Can you work these out from the model? Positions are in its coordinate system, mm. A direction names the side the tool comes from. Round coordinates to 2 decimals unless told otherwise and drop trailing zeros. Order: outer loops, then holes, each group sorted by start corner. A loop starts at its lowest first (then second) coordinate and runs counter-clockwise, first axis right, second up. Notation, with made-up numbers: (89, -27.5) -> (141, -27.5) arc R15 cw to (141, -15.5) -> close; hole circle Ø3 at (55.5, 47.5). An arc over 180 degrees is marked (long way). Use a Markdown table: item, result. Add a question column.
Q1. If we section it at A-A on y = 0: Give the number of separate pieces and of enclosed holes in the cut face, plus the area to 3 significant figures.
Q2. I'm going to push flat-ended pins straight in: pin 1 Ø3 at (y, z) = (2.5, 10) entering from +X; pin 2 Ø2 at (x, z) = (-7, 4) entering from +Y; pin 3 Ø5 at (x, z) = (-4, 11.5) entering from +Y; pin 4 Ø3 at (x, y) = (9, 0) entering from -Z. Where does each tip first touch, or does it pass through?
Q3. I need wall thicknesses on line 1 along Y through (x, z) = (9, 12.9); line 2 along Y through (x, z) = (-1.5, 13); line 3 along Z through (x, y) = (-8, -7). Which ranges of each line are inside material? Lowest first, please. Write a range as [from, to].
Q4. We'd pull the mould along Z, two halves only. Please class faces 3 (the face through (8.77, -19.67, 3.04)), 4 (the face through (0, -5, 0)), 5 (the face through (7, 0, 12)), 6 (the face through (0, 10, 10)): +Z half, -Z half, draft (parallel to the pull), parting line (faces both ways), or undercut.
Q5. For faces 1 (the face through (15.63, 0.14, 11.56)), 2 (the face through (6.2, 0, 11)), which set-ups out of +Z, -Z, +X, -X, +Y, -Y let a thin tool reach every point of the face, with its end or its side?
Q6. If we section it at B-B on y = 6: List the corners of the cut face in (x, z) for me.
```python
from build123d import *

# Parameters (mm, degrees)
ESBO_O1_W                = 34.6
ESBO_O1_H                = 26
RESSALTO_EXTRUS_O1_DEPTH = 7
ESBO_O10_W               = 34.6
ESBO_O10_H               = 2.5
RESSALTO_EXTRUS_O4_DEPTH = 7
CHANFRO1_SIZE            = 7
CHANFRO2_SIZE2           = 7
CHANFRO2_SIZE            = 2.54779164
ESBO_O11_W               = 5.6
ESBO_O11_H               = 3
RESSALTO_EXTRUS_O5_DEPTH = 10
ESBO_O12_R               = 1.75
CORTE_EXTRUS_O1_DEPTH    = 20
ESBO_O13_W               = 34.6
ESBO_O13_H               = 5.5
ESBO_O13_H_2             = 18.393079324
CORTE_EXTRUS_O2_DEPTH    = 1


with BuildPart() as part:
    # Esboço1 → Ressalto-extrusão1 (new body)
    with BuildSketch(Plane.XY):
        Rectangle(ESBO_O1_W, ESBO_O1_H)
    extrude(amount=RESSALTO_EXTRUS_O1_DEPTH)

    # Esboço10 → Ressalto-extrusão4 (add)
    with BuildSketch(Plane(origin=(0, 0, 0), x_dir=(-1, 0, 0), z_dir=(0, 0, -1))):
        Polygon((-17.3, -19.5), (0, -26.5), (17.3, -19.5), (17.3, -13), (-17.3, -13), align=None)
        with Locations((0, 14.25)):
            Rectangle(ESBO_O10_W, ESBO_O10_H)
    extrude(amount=-RESSALTO_EXTRUS_O4_DEPTH)

    # Chanfro1
    chanfro1_edges = [part.edges().sort_by_distance(p)[0] for p in [
        (8.65, -23, 7),
        (-8.65, -23, 7),
    ]]
    chamfer(chanfro1_edges, length=CHANFRO1_SIZE - 0.0001)  # a hair under: the kernel refuses the full size

    # Chanfro2
    chanfro2_edges = [part.edges().sort_by_distance(p)[0] for p in [
        (0, 15.5, 7),
    ]]
    chanfro2_side = [part.faces().sort_by_distance(p)[0] for p in [
        (0, 15.449044167, 7),
    ]]
    chamfer(chanfro2_edges, length=CHANFRO2_SIZE - 0.0001, length2=CHANFRO2_SIZE2 - 0.0001, reference=chanfro2_side[0])  # a hair under: the kernel refuses the full size

    # Esboço11 → Ressalto-extrusão5 (add, symmetric)
    with BuildSketch(Plane(origin=(0, 0, 0), x_dir=(1, 0, 0), z_dir=(0, 1, 0))):
        with BuildLine():
            Line((-17.3, -7), (-14, -16))
            Line((-14, -16), (-5.196152423, -16))
            ThreePointArc((-5.196152423, -16), (0, -13), (5.196152423, -16))
            Line((5.196152423, -16), (14, -16))
            Line((14, -16), (17.3, -7))
            Line((17.3, -7), (-17.3, -7))
        make_face()
        with Locations((-9, -10.5)):
            Rectangle(ESBO_O11_W, ESBO_O11_H, mode=Mode.SUBTRACT)
        with Locations((9, -10.5)):
            Rectangle(ESBO_O11_W, ESBO_O11_H, mode=Mode.SUBTRACT)
    extrude(amount=RESSALTO_EXTRUS_O5_DEPTH, both=True)

    # Esboço12 → Corte-extrusão1 (cut)
    with BuildSketch(Plane.XY.offset(16)):
        with Locations((-9, 0)):
            Circle(ESBO_O12_R)
        with Locations(Location((9, 0, 0), (0, 0, 180))):
            Circle(ESBO_O12_R)
    extrude(amount=-CORTE_EXTRUS_O1_DEPTH, mode=Mode.SUBTRACT)

    # Esboço13 → Corte-extrusão2 (cut)
    with BuildSketch(Plane.XY.offset(7)):
        with Locations((0, 12.75)):
            Rectangle(ESBO_O13_W, ESBO_O13_H)
        with Locations((0, -19.196539662)):
            Rectangle(ESBO_O13_W, ESBO_O13_H_2)
    extrude(amount=-CORTE_EXTRUS_O2_DEPTH, mode=Mode.SUBTRACT)


solid = part.part
```
Answer below:
| question | item | result |
|---|---|---|
| 1 | separate pieces | 3 |
| 1 | enclosed holes | 0 |
| 1 | area | 377 mm² |
| 2 | pin 1 | x = 16.75 |
| 2 | pin 2 | y = 14.41 |
| 2 | pin 3 | y = 10 |
| 2 | pin 4 | through |
| 3 | line 1 | [-10, -1.75], [1.75, 10] |
| 3 | line 2 | [-10, 10] |
| 3 | line 3 | [0, 9], [12, 16] |
| 4 | face 3 | +Z half |
| 4 | face 4 | -Z half |
| 4 | face 5 | undercut |
| 4 | face 6 | draft |
| 5 | face 1 | +Z, +X, +Y, -Y |
| 5 | face 2 | +Y, -Y |
| 6 | outline | (-17.3, 0) -> (17.3, 0) -> (17.3, 7) -> (14, 16) -> (5.2, 16) arc R6 cw to (-5.2, 16) -> (-14, 16) -> (-17.3, 7) -> close; hole (-11.8, 9) -> (-6.2, 9) -> (-6.2, 12) -> (-11.8, 12) -> close; hole (6.2, 9) -> (11.8, 9) -> (11.8, 12) -> (6.2, 12) -> close |
